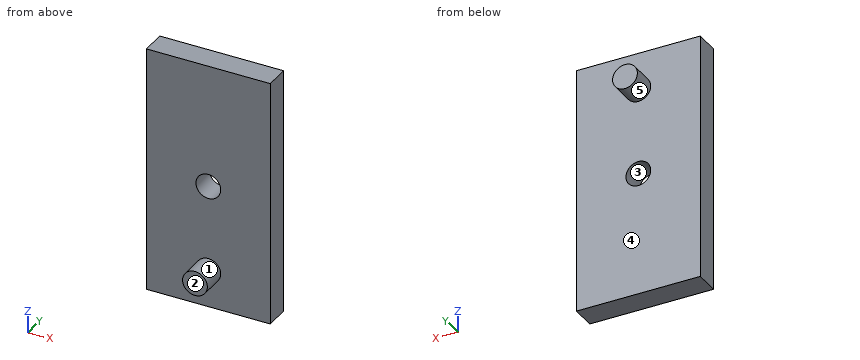
```python
from build123d import *

# Parameters (mm, degrees)
F0_W     = 100
F0_H     = 200
F1_DEPTH = 20
F2_R     = 10
F3_DEPTH = 20.001
F4_R     = 10
F5_DEPTH = 20
F6_R     = 10
F7_DEPTH = 20


with BuildPart() as f1:
    # F0 (on Front) → F1 (new body)
    with BuildSketch(Plane.XZ):
        Rectangle(F0_W, F0_H)
    extrude(amount=F1_DEPTH)

    # F2 (on face) → F3 (cut, through all)
    with BuildSketch(Plane.XZ.offset(20)):
        Circle(F2_R)
    extrude(amount=-F3_DEPTH, mode=Mode.SUBTRACT)

    # F4 (on face) → F5 (join)
    with BuildSketch(Plane.XZ.offset(20)):
        with Locations((0, -70)):
            Circle(F4_R)
    extrude(amount=F5_DEPTH)

    # F6 (on face) → F7 (join)
    with BuildSketch(Plane(origin=(0, 0, 0), x_dir=(-1, 0, 0), z_dir=(0, 1, 0))):
        with Locations((0, 70)):
            Circle(F6_R)
    extrude(amount=F7_DEPTH)


solid = f1.part
```
For this review, take the finished solid that the model builds, in its own axes (mm). Face numbers are marked on the shaded views. A direction names the side the tool comes from. Round coordinates to 2 decimals unless told otherwise and drop trailing zeros. Write each loop counter-clockwise with the first axis right and the second up, starting at its lowest first coordinate (ties: lowest second). Pieces come first, ordered by that corner, then holes. Notation, with made-up numbers: (41.25, 19) - (55.25, 19) arc R18 ccw to (55.25, 45) - close; hole circle Ø4 at (32, 6.25). An arc over 180 degrees is marked (long way). Put each result on its own line as item: value.
Q1. Machinability: for the marked faces 1 and 2, which of the approach directions +Z, -Z, +X, -X, +Y, -Y give a long, thin tool a straight path to every point of the face, cutting with its end or side? Answer none if there is none.
Solved:
face 1: -Y
face 2: +Z, -Z, +X, -X, -Y
Q2. Insertion check: pin 1 Ø8 at (x, z) = (30, -52) entering from +Y. The pin has a flat end and moves straight along its axis. Give the tip position at first contact, or say it passes through.
Solved:
pin 1: stops at y = 0
Q3. We need section A-A (z = 0). Give the boundary of the cut face in (x, y), and give its area (3 significant figures).
Solved:
outline: (-50, -20) - (-10, -20) - (-10, 0) - (-50, 0) - close; (10, -20) - (50, -20) - (50, 0) - (10, 0) - close
area: 1,600 mm2
Q4. Mouldability with a two-part tool opening along Z and no side actions: class the marked faces 3, 4 and 5 as released by +Z, released by -Z, zero draft, split by the parting line, or undercut.
Solved:
face 3: undercut
face 4: zero draft
face 5: split by the parting line
Q5. We need section B-B (x = 0). Give the boundary of the cut face in (y, z), and give its area (3 significant figures).
Solved:
outline: (-40, -80) - (-20, -80) - (-20, -100) - (0, -100) - (0, -10) - (-20, -10) - (-20, -60) - (-40, -60) - close; (-20, 10) - (0, 10) - (0, 60) - (20, 60) - (20, 80) - (0, 80) - (0, 100) - (-20, 100) - close
area: 4,400 mm2
Q6. Wall thickness on probe 1 along Z at (x, y) = (0, -10); probe 2 along Y at (x, z) = (-22.5, -23.5); probe 3 along Y at (x, z) = (-1.5, 70): over which ranges is each line inside the solid? List them lowest first.
Solved:
probe 1: z = -100 to -10, 10 to 100
probe 2: y = -20 to 0
probe 3: y = -20 to 20
Q7. We need section C-C (y = -11.5). Give the boundary of the cut face in (x, z), and give its area (3 significant figures).
Solved:
outline: (-50, -100) - (50, -100) - (50, 100) - (-50, 100) - close; hole circle Ø20 at (0, 0)
area: 19,700 mm2
Q8. We need section D-D (z = 70). Give the boundary of the cut face in (x, y).
Solved:
outline: (-50, -20) - (50, -20) - (50, 0) - (10, 0) - (10, 20) - (-10, 20) - (-10, 0) - (-50, 0) - close
